from build123d import *

# Parameters (mm, degrees)
SKETCH1_W           = 200
SKETCH1_H           = 120
SKETCH1_W_2         = 160
SKETCH1_H_2         = 80
BOSS_EXTRUDE1_DEPTH = 3.1
SKETCH2_W           = 100
SKETCH2_H           = 3.1
BOSS_EXTRUDE2_DEPTH = 3.1
FILLET1_R           = 35


with BuildPart() as part:
    # Sketch1 → Boss-Extrude1 (new body)
    with BuildSketch(Plane.XY):
        Rectangle(SKETCH1_W, SKETCH1_H)
        Rectangle(SKETCH1_W_2, SKETCH1_H_2, mode=Mode.SUBTRACT)
    extrude(amount=BOSS_EXTRUDE1_DEPTH)

    # Sketch2 → Boss-Extrude2 (add)
    with BuildSketch(Plane.XY.offset(3.1)):
        with Locations((0, 61.55)):
            Rectangle(SKETCH2_W, SKETCH2_H)
        with Locations((0, -61.55)):
            Rectangle(SKETCH2_W, SKETCH2_H)
    extrude(amount=-BOSS_EXTRUDE2_DEPTH)

    # Fillet1
    fillet1_edges = [part.edges().sort_by_distance(p)[0] for p in [
        (80, -40, 1.55),
        (80, 40, 1.55),
        (-80, 40, 1.55),
        (-80, -40, 1.55),
    ]]
    fillet(fillet1_edges, radius=FILLET1_R)


solid = part.part
Read the model definition and answer for the solid it produces. Units are mm, in the model's axes. A direction names the side the tool comes from. Round coordinates to 2 decimals unless told otherwise and drop trailing zeros. Write each loop counter-clockwise with the first axis right and the second up, starting at its lowest first coordinate (ties: lowest second). Pieces come first, ordered by that corner, then holes. Notation, with made-up numbers: (22, 84) - (78, 84) arc R27 cw to (78, 106) - close; hole circle Ø5 at (55, 38.5). An arc over 180 degrees is marked (long way). Use a Markdown table: item, result.
(1) Each of these flat-tipped pins is pushed along its axis until it touches: pin 1 Ø0.9 at (x, z) = (-64.5, 2.5) entering from -Y; pin 2 Ø1.5 at (y, z) = (62, 1) entering from -X; pin 3 Ø1.5 at (y, z) = (62, 2) entering from +X. Where does it stop, or does it pass through?
Reported:
| item | result |
|---|---|
| pin 1 | y = -60 |
| pin 2 | x = -50 |
| pin 3 | x = 50 |
(2) Which of the six approach directions +Z, -Z, +X, -X, +Y, -Y give full straight-line access (tool end or side, diameter ignored) to faces 4 (the cylindrical face through (-69.475, 30.019, 1.572)), 5 (the flat face through (-1, 43, 3.1))?
Reported:
| item | result |
|---|---|
| face 4 | +Z, -Z |
| face 5 | +Z, +X, -X, +Y, -Y |
(3) The part is cut by section C-C (y = 2). Write down the section's boundary in (x, z).
Reported:
| item | result |
|---|---|
| outline | (-100, 0) - (-80, 0) - (-80, 3.1) - (-100, 3.1) - close; (80, 0) - (100, 0) - (100, 3.1) - (80, 3.1) - close |
(4) The part is cut by section A-A (z = 1.15). Write down the section's boundary in (x, y).
Reported:
| item | result |
|---|---|
| outline | (-100, -60) - (-50, -60) - (-50, -63.1) - (50, -63.1) - (50, -60) - (100, -60) - (100, 60) - (50, 60) - (50, 63.1) - (-50, 63.1) - (-50, 60) - (-100, 60) - close; hole (-80, -5) arc R35 ccw to (-45, -40) - (45, -40) arc R35 ccw to (80, -5) - (80, 5) arc R35 ccw to (45, 40) - (-45, 40) arc R35 ccw to (-80, 5) - close |
(5) Straight lines are drawn through the part: line 1 along Y through (x, z) = (-12, 2.6); line 2 along X through (y, z) = (0.5, 0.4); line 3 along Y through (x, z) = (55.5, 2.35). For each, find the intervals that lie inside material, in ascending order. Write a range as [from, to].
Reported:
| item | result |
|---|---|
| line 1 | [-63.1, -40], [40, 63.1] |
| line 2 | [-100, -80], [80, 100] |
| line 3 | [-60, -38.39], [38.39, 60] |
(6) The part is cut by section B-B (x = -73). Write down the section's boundary in (y, z), then the cut area to 3 significant figures.
Reported:
| item | result |
|---|---|
| outline | (-60, 0) - (-26, 0) - (-26, 3.1) - (-60, 3.1) - close; (26, 0) - (60, 0) - (60, 3.1) - (26, 3.1) - close |
| area | 211 mm2 |
(7) The mould has two halves that part along Y. Classify faces 1 (the cylindrical face through (-69.475, -30.019, 1.572)), 2 (the flat face through (-1, 43, 0)), 3 (the cylindrical face through (69.475, -30.019, 1.572)): released by +Y, released by -Y, zero draft, split by the parting line, or undercut.
Reported:
| item | result |
|---|---|
| face 1 | undercut |
| face 2 | zero draft |
| face 3 | undercut |
